from build123d import *

# Parameters (mm, degrees)
BASE_FLANGE1_DEPTH = 10
SKETCH6_R          = 1.984375
CUT_EXTRUDE1_DEPTH = 10
SKETCH7_R          = 1.984375
CUT_EXTRUDE2_DEPTH = 59.480991085


# Sheet-metal steps are written as plain solids
with BuildPart() as part:
    # Sketch1 → Base-Flange1 (new body)
    with BuildSketch(Plane(origin=(0, 0, 0), x_dir=(1, 0, 0), z_dir=(0, 1, 0))):
        with BuildLine():
            Line((0, 40), (0, 0.7366))
            ThreePointArc((0, 0.7366), (0.215745145, 0.215745145), (0.7366, 0))
            Line((0.7366, 0), (39.2634, 0))
            ThreePointArc((39.2634, 0), (39.784254855, 0.215745145), (40, 0.7366))
            Line((40, 0.7366), (40, 40))
            Line((40, 40), (40.7366, 40))
            Line((40.7366, 40), (40.7366, 0.7366))
            ThreePointArc((40.7366, 0.7366), (40.30510971, -0.30510971), (39.2634, -0.7366))
            Line((39.2634, -0.7366), (0.7366, -0.7366))
            ThreePointArc((0.7366, -0.7366), (-0.30510971, -0.30510971), (-0.7366, 0.7366))
            Line((-0.7366, 0.7366), (-0.7366, 40))
            Line((-0.7366, 40), (0, 40))
        make_face()
    extrude(amount=BASE_FLANGE1_DEPTH)

    # Sketch6 → Cut-Extrude1 (cut)
    with BuildSketch(Plane.XY.offset(0.7366)):
        with Locations((5.7366, 5)):
            Circle(SKETCH6_R)
        with Locations((34.2634, 5)):
            Circle(SKETCH6_R)
    extrude(amount=-CUT_EXTRUDE1_DEPTH, mode=Mode.SUBTRACT)

    # Sketch7 → Cut-Extrude2 (cut, through all)
    with BuildSketch(Plane.ZY.offset(0.7366)):
        with Locations((-35, 5)):
            Circle(SKETCH7_R)
    extrude(amount=-CUT_EXTRUDE2_DEPTH, mode=Mode.SUBTRACT)


solid = part.part
Source: CAD feature listing. Evaluate the final solid. Frame: model axes, mm. A direction names the side the tool comes from. Round coordinates to 2 decimals unless told otherwise and drop trailing zeros. Loops run counter-clockwise (first coordinate to the right, second up) from the corner with the lowest first, then second, coordinate; pieces in that order, holes last.
Q1. Section A-A, the plane z = -14.5. Return loops of the section in (x, y), plus the area to 3 significant figures.
Q2. Section C-C, the plane z = -35. Return loops of the section in (x, y), plus the area to 3 significant figures.
Q3. Section B-B, the plane y = 5. Return loops of the section in (x, z).
Q4. Section D-D, the plane x = 5.5. Return loops of the section in (y, z), plus the area to 3 significant figures.
Q5. Access query for faces 5 (the face through (0, 5, -21)), 6 (the face through (35.33, 6.673, 0.373)). Directions: +Z, -Z, +X, -X, +Y, -Y. A direction counts if a zero-diameter tool reaches every point of the face in a straight line with its end or side. Return the directions, or none.
Q6. First-contact query: P1, Ø2.5, axis at y = 5, z = -35, coming from the +X side; P2, Ø6, axis at x = 28, y = 4.5, coming from the -Z side. Flat tips, straight axial feed; report the tip coordinate or a pass-through.
Q7. Ray query, line 1 (X direction, y = 6.5, z = -21); line 2 (Z direction, x = 17, y = 3). Return the intervals inside material, ascending.
Q8. Mould query, pull axis Z, two halves, no side actions, for faces 1 (the face through (20, 5, 0)), 2 (the face through (40.737, 5, -21)), 3 (the face through (20, 5, 0.737)), 4 (the face through (40.36, 6.67, -33.93)). Classes: pulls with the +Z half, pulls with the -Z half, needs draft (parallel to the pull), parting line crosses it, or undercut.
Solutions:
1. outline: (-0.74, 0) - (0, 0) - (0, 10) - (-0.74, 10) - close; (40, 0) - (40.74, 0) - (40.74, 10) - (40, 10) - close
1. area: 14.7 mm2
2. outline: (-0.74, 0) - (0, 0) - (0, 3.02) - (-0.74, 3.02) - close; (-0.74, 6.98) - (0, 6.98) - (0, 10) - (-0.74, 10) - close; (40, 0) - (40.74, 0) - (40.74, 3.02) - (40, 3.02) - close; (40, 6.98) - (40.74, 6.98) - (40.74, 10) - (40, 10) - close
2. area: 8.89 mm2
3. outline: (-0.74, -40) - (0, -40) - (0, -36.98) - (-0.74, -36.98) - close; (-0.74, -33.02) - (0, -33.02) - (0, -0.74) arc R0.74 cw to (0.74, 0) - (3.75, 0) - (3.75, 0.74) - (0.74, 0.74) arc R1.47 ccw to (-0.74, -0.74) - close; (7.72, 0) - (32.28, 0) - (32.28, 0.74) - (7.72, 0.74) - close; (36.25, 0) - (39.26, 0) arc R0.74 cw to (40, -0.74) - (40, -33.02) - (40.74, -33.02) - (40.74, -0.74) arc R1.47 ccw to (39.26, 0.74) - (36.25, 0.74) - close; (40, -40) - (40.74, -40) - (40.74, -36.98) - (40, -36.98) - close
4. outline: (0, 0) - (3.03, 0) - (3.03, 0.74) - (0, 0.74) - close; (6.97, 0) - (10, 0) - (10, 0.74) - (6.97, 0.74) - close
4. area: 4.46 mm2
5. face 5: -Z, +Y, -Y
5. face 6: +Z, -Z
6. P1: passes through
6. P2: stops at z = 0
7. line 1: x = -0.74 to 0, 40 to 40.74
7. line 2: z = 0 to 0.74
8. face 1: pulls with the -Z half
8. face 2: needs draft
8. face 3: pulls with the +Z half
8. face 4: undercut
